Geometry check sheet. Reference: drawing and pictorial views, mm from the part's lowest x, y, z. A direction names the side the tool comes from. Coordinates: 2 decimals unless noted, no trailing zeros. Write each loop counter-clockwise with the first axis right and the second up, starting at its lowest first coordinate (ties: lowest second). Pieces come first, ordered by that corner, then holes. Notation, with made-up numbers: (5, -1) - (38, -1) arc R17 cw to (38, 30) - close; hole circle Ø11 at (50.25, -12). An arc over 180 degrees is marked (long way). Answer as CSV lines item,"result". Start each with the question number.
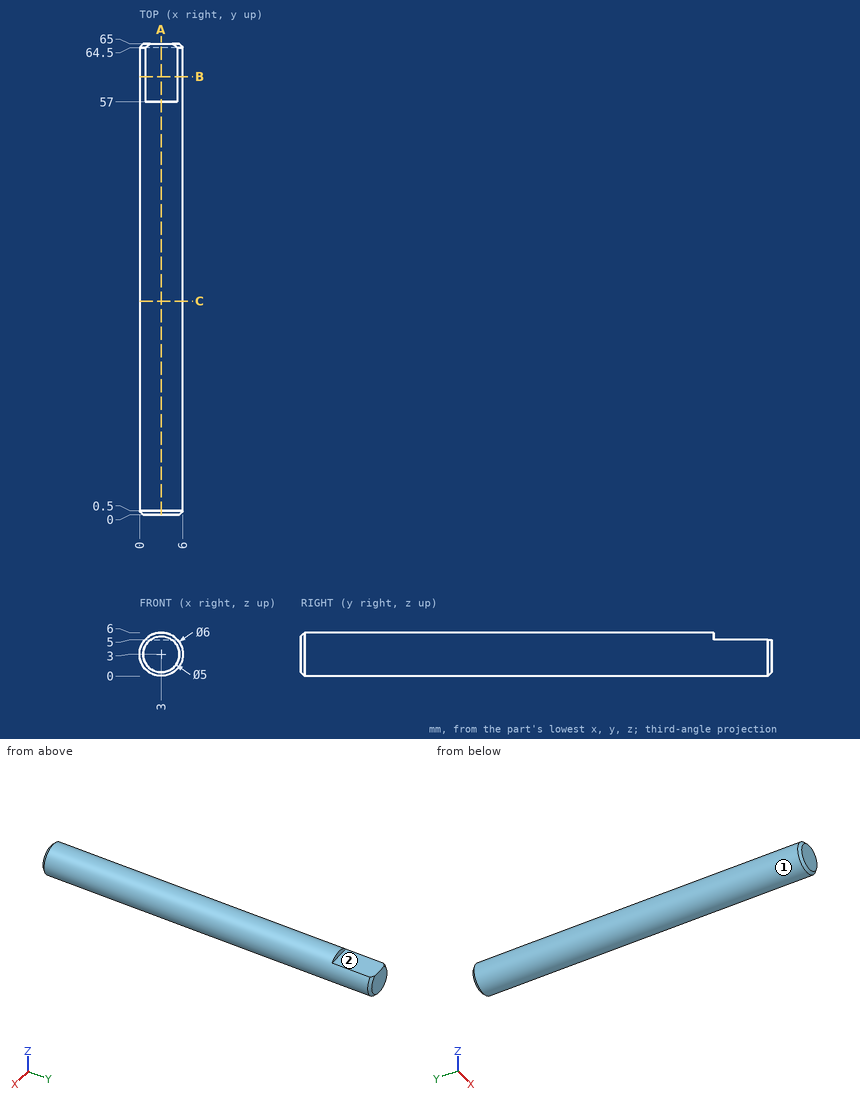
1. Scan lines: line 1 along Z through (x, y) = (2.8, 40); line 2 along Y through (x, z) = (4.05, 0.6). Record each from-to range of solid material in increasing order. Write a range as from..to.
2. Cross-section at B-B (y = 60.5). Record the cut outline in (x, z), and give its area (3 significant figures).
3. Cross-section at C-C (y = 29.5). Record the cut outline in (x, z).
4. Access from +Z, -Z, +X, -X, +Y, -Y to the whole of each face (thin tool, end or side, straight path). Record for the marked faces 1 and 2.
5. Depth check by flat-ended pin: P1, Ø1.5, axis at x = 2, y = 18.5, coming from the +Z side; P2, Ø0.8, axis at x = 3.5, z = 5.5, coming from the +Y side; P3, Ø1, axis at x = 1, y = 8, coming from the -Z side. Enter the tip coordinate at first touch or a pass-through.
6. Cross-section at A-A (x = 3). Record the cut outline in (y, z), and give its area (3 significant figures).
Completed:
1,line 1,"z = 0.01..5.99"
1,line 2,"y = 0.12..64.88"
2,outline,"(0.76, 5) arc R3 ccw (long way) to (5.24, 5) - close"
2,area,"25.2 mm2"
3,outline,"circle Ø6 at (3, 3)"
4,face 1,"+Y, -Y"
4,face 2,"+Z, +X, -X, +Y"
5,P1,"stops at z = 5.99"
5,P2,"stops at y = 57"
5,P3,"stops at z = 0.4"
6,outline,"(0, 0.5) - (0.5, 0) - (64.5, 0) - (65, 0.5) - (65, 5) - (57, 5) - (57, 6) - (0.5, 6) - (0, 5.5) - close"
6,area,"382 mm2"
